Model file for the job. Use its own axes, mm. Face numbers are marked on the shaded views. Give positions to 0.01 mm unless a question says otherwise; leave off trailing zeros. Order: outer loops, then holes, each group sorted by start corner. A loop starts at its lowest first (then second) coordinate and runs counter-clockwise, first axis right, second up. Notation, with made-up numbers: (65, 42.25) -> (117, 42.25) arc R19 cw to (117, 58.25) -> close; hole circle Ø1 at (37, -33.75). An arc over 180 degrees is marked (long way). Use CSV: the item, a comma, the result in double quotes. Start each with the question number.
1. Wall check: line 1 (X direction, y = 4.75, z = 1.27) (3 decimals); line 2 (X direction, y = 6.25, z = -12.5); line 3 (Z direction, x = 11, y = 3.75). Give the ranges that are in metal, low to high. Write a range as from..to.
2. Cut at C-C on x = -2. List the corners of the cut face in (y, z), then the cut area to 3 significant figures.
3. Cut at B-B on y = 5.5. Give the number of separate pieces and of enclosed holes in the cut face, then the cut area to 3 significant figures.
4. Cut at A-A on z = 1.5. List the corners of the cut face in (x, y), then the cut area to 3 significant figures.
5. Pull direction Z, two halves, no side cores. Call the marked faces 1, 2, 3 and 4: released by +Z, released by -Z, zero draft, split by the parting line, or undercut.
6. Cut at D-D on x = -26.5. List the corners of the cut face in (y, z), then the cut area to 3 significant figures.
7. Drop flat-ended pins along their axis: pin 1 (5 mm diameter, centred on x = 0, z = -25.146, fed in from +Y); pin 2 (2 mm diameter, centred on x = 16.5, y = 4, fed in from +Z); pin 3 (10 mm diameter, centred on x = 0, z = -4.826, fed in from +Y); pin 4 (2 mm diameter, centred on y = 3.5, z = 7.5, fed in from -X). Give the stop position or say it passes through.
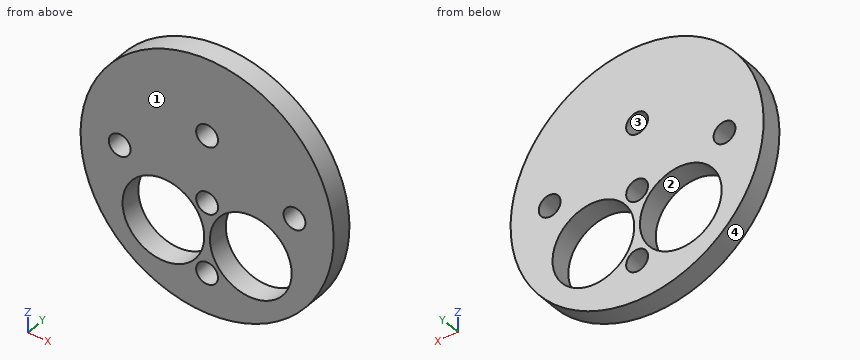
```python
from build123d import *

# Parameters (mm, degrees)
SKETCH1_W               = 36.7665
SKETCH1_H               = 6.35
CUT_EXTRUDE1_DEPTH      = 53.381996378
CUT_EXTRUDE1_DEPTH_BACK = 53.381996378
SKETCH2_R               = 11.8745
SKETCH2_R_2             = 3.175
CUT_EXTRUDE2_DEPTH      = 53.381996378
CUT_EXTRUDE2_DEPTH_BACK = 53.381996378
SKETCH3_R               = 3.175


with BuildPart() as part:
    # Sketch1 → Revolve1 (revolve)
    with BuildSketch(Plane.XY, mode=Mode.PRIVATE) as revolve1_sk:
        with Locations((18.38325, 3.175)):
            Rectangle(SKETCH1_W, SKETCH1_H)
    revolve(revolve1_sk.sketch.rotate(Axis((0, 0, 0), (0, 1, 0)), 90), axis=Axis((0, 0, 0), (0, 1, 0)))

    # Sketch2 → Cut-Extrude1 (cut, two sides: drawn at the far end of the back side and taken through both)
    with BuildSketch(Plane(origin=(0, 6.35, 0), x_dir=(1, 0, 0), z_dir=(0, 1, 0)).offset(-CUT_EXTRUDE1_DEPTH_BACK)):
        with Locations(Location((-12.7, 14.986, 0), (0, 0, 270))):
            Circle(SKETCH2_R)
        with Locations(Location((12.7, 14.986, 0), (0, 0, 270))):
            Circle(SKETCH2_R)
        with Locations(Location((0, 25.146, 0), (0, 0, 270))):
            Circle(SKETCH2_R_2)
        with Locations(Location((0, 4.826, 0), (0, 0, 270))):
            Circle(SKETCH2_R_2)
        with Locations(Location((0, -14.605, 0), (0, 0, 270))):
            Circle(SKETCH2_R_2)
    extrude(amount=CUT_EXTRUDE1_DEPTH + CUT_EXTRUDE1_DEPTH_BACK, mode=Mode.SUBTRACT)

    # Sketch3 → Cut-Extrude2 (cut, two sides: drawn at the far end of the back side and taken through both)
    with BuildSketch(Plane(origin=(0, 6.35, 0), x_dir=(1, 0, 0), z_dir=(0, 1, 0)).offset(-CUT_EXTRUDE2_DEPTH_BACK)):
        with Locations(Location((-25.4, -1.27, 0), (0, 0, 270))):
            Circle(SKETCH3_R)
        with Locations(Location((25.4, -1.27, 0), (0, 0, 270))):
            Circle(SKETCH3_R)
    extrude(amount=CUT_EXTRUDE2_DEPTH + CUT_EXTRUDE2_DEPTH_BACK, mode=Mode.SUBTRACT)


solid = part.part
```
Verdict:
1,line 1,"-36.745..-28.575, -22.225..22.225, 28.575..36.745"
1,line 2,"-34.58..-24.31, -1.09..1.09, 24.31..34.58"
1,line 3,"-35.08..-26.74, -3.23..35.08"
2,outline,"(0, -36.71) -> (6.35, -36.71) -> (6.35, -27.61) -> (0, -27.61) -> close; (0, -22.68) -> (6.35, -22.68) -> (6.35, -20.14) -> (0, -20.14) -> close; (0, -9.84) -> (6.35, -9.84) -> (6.35, -7.29) -> (0, -7.29) -> close; (0, -2.36) -> (6.35, -2.36) -> (6.35, 12.14) -> (0, 12.14) -> close; (0, 17.07) -> (6.35, 17.07) -> (6.35, 36.71) -> (0, 36.71) -> close"
2,area,"307 mm^2"
3,separate pieces,"1"
3,enclosed holes,"7"
3,area,"3,200 mm^2"
4,outline,"(-36.74, 0) -> (-28.57, 0) -> (-28.57, 6.35) -> (-36.74, 6.35) -> close; (-22.23, 0) -> (22.23, 0) -> (22.23, 6.35) -> (-22.23, 6.35) -> close; (28.57, 0) -> (36.74, 0) -> (36.74, 6.35) -> (28.57, 6.35) -> close"
4,area,"386 mm^2"
5,face 1,"zero draft"
5,face 2,"undercut"
5,face 3,"undercut"
5,face 4,"split by the parting line"
6,outline,"(0, -25.49) -> (6.35, -25.49) -> (6.35, -1.71) -> (0, -1.71) -> close; (0, 4.25) -> (6.35, 4.25) -> (6.35, 25.49) -> (0, 25.49) -> close"
6,area,"286 mm^2"
7,pin 1,"through"
7,pin 2,"z = 33.34"
7,pin 3,"y = 6.35"
7,pin 4,"x = -36.19"
